Read the model definition and answer for the solid it produces. Units are mm, in the model's axes. A direction names the side the tool comes from. Coordinates: 2 decimals unless noted, no trailing zeros. Write each loop counter-clockwise with the first axis right and the second up, starting at its lowest first coordinate (ties: lowest second). Pieces come first, ordered by that corner, then holes.
Item 1: Straight lines are drawn through the part: probe 1 along X at (y, z) = (2.45, -253); probe 2 along X at (y, z) = (2.3, -255); probe 3 along X at (y, z) = (2.4, -228.5). For each, find the intervals that lie inside material, in ascending order.
Item 2: A tool of negligible diameter and unlimited length cuts with its end or side. For faces 4 (the face through (252.034, 2, -201)), 5 (the face through (247, 3.175, -240)), from which of +Z, -Z, +X, -X, +Y, -Y can it reach the whole face along a straight path? Write none if from no direction.
Item 3: Determine the mould class of faces 1 (the face through (240, 2, -269.211)), 2 (the face through (265, 2, -193.011)), 3 (the face through (236.533, 2.976, -253.457)) for opening direction Z: released by +Z, released by -Z, zero draft, split by the parting line, or undercut.
Item 4: Section C-C (x = 230) is taken. Give the vertices of the cut face in (y, z) (3 decimals), then the cut area to 3 significant figures.
Item 5: Section B-B (x = 262) is taken. State how many separate pieces and enclosed holes the cut face has, then the cut area to 3 significant figures.
Item 6: Section A-A (y = 1.35) is taken. Give the vertices of the cut face in (x, z).
Item 7: This flat-tipped pin is pushed along its axis until it touches: P1, Ø8, axis at x = 253.5, z = -215, coming from the -Y side. Where does it stop, or does it pass through?
from build123d import *

# Parameters (mm, degrees)
BOSS_EXTRUDE1_DEPTH                  = 3.175
F_1_4_0_25_DIAMETER_HOLE1_AT_2_COUNT = 2
F_1_4_0_25_DIAMETER_HOLE1_AT_2_PITCH = 25.4
F_1_4_0_25_DIAMETER_HOLE1_AT_3_COUNT = 2
F_1_4_0_25_DIAMETER_HOLE1_AT_3_PITCH = 50.8
F_1_4_0_25_DIAMETER_HOLE1_AT_4_COUNT = 2
F_1_4_0_25_DIAMETER_HOLE1_AT_4_PITCH = 56.796126628
F_1_4_0_25_DIAMETER_HOLE1_AT_5_COUNT = 2
F_1_4_0_25_DIAMETER_HOLE1_AT_5_PITCH = 71.842048969


with BuildPart() as part:
    # Sketch1 → Boss-Extrude1 (new body)
    with BuildSketch(Plane(origin=(0, 0, 0), x_dir=(1, 0, 0), z_dir=(0, 1, 0))):
        with BuildLine():
            Line((274.893771244, 269.21115375), (203.773771244, 269.21115375))
            ThreePointArc((203.773771244, 269.21115375), (201.97772002, 268.467204975), (201.233771244, 266.67115375))
            Line((201.233771244, 266.67115375), (201.233771244, 246.35115375))
            ThreePointArc((201.233771244, 246.35115375), (201.97772002, 244.555102526), (203.773771244, 243.81115375))
            Line((203.773771244, 243.81115375), (213.933771244, 243.81115375))
            ThreePointArc((213.933771244, 243.81115375), (240.874539608, 232.651922114), (252.033771244, 205.71115375))
            Line((252.033771244, 205.71115375), (252.033771244, 195.55115375))
            ThreePointArc((252.033771244, 195.55115375), (252.77772002, 193.755102526), (254.573771244, 193.01115375))
            Line((254.573771244, 193.01115375), (274.893771244, 193.01115375))
            ThreePointArc((274.893771244, 193.01115375), (276.689822469, 193.755102526), (277.433771244, 195.55115375))
            Line((277.433771244, 195.55115375), (277.433771244, 266.67115375))
            ThreePointArc((277.433771244, 266.67115375), (276.689822469, 268.467204975), (274.893771244, 269.21115375))
        make_face()
    extrude(amount=BOSS_EXTRUDE1_DEPTH)

    # Sketch4 → 1/4 (0.25) Diameter Hole1 (revolve, cut)
    with BuildSketch(Plane(origin=(264.733771244, 0, -205.71115375), x_dir=(0, 0, -1), z_dir=(1, 0, 0))):
        Polygon((0, 0), (0, 3.175), (3.175, 3.175), (3.175, 4.090710056), (6.731, 0), align=None)
    f_1_4_0_25_diameter_hole1 = revolve(axis=Axis((264.733771244, -6.35, -205.71115375), (0, 1, 0)), mode=Mode.SUBTRACT)

    # 1/4 (0.25) Diameter Hole1 at 2: 1/4 (0.25) Diameter Hole1 ×2
    with Locations(*[(0, 0, -i * F_1_4_0_25_DIAMETER_HOLE1_AT_2_PITCH) for i in range(1, F_1_4_0_25_DIAMETER_HOLE1_AT_2_COUNT)]):
        add(f_1_4_0_25_diameter_hole1, mode=Mode.SUBTRACT)

    # 1/4 (0.25) Diameter Hole1 at 3: 1/4 (0.25) Diameter Hole1 ×2
    with Locations(*[(0, 0, -i * F_1_4_0_25_DIAMETER_HOLE1_AT_3_PITCH) for i in range(1, F_1_4_0_25_DIAMETER_HOLE1_AT_3_COUNT)]):
        add(f_1_4_0_25_diameter_hole1, mode=Mode.SUBTRACT)

    # 1/4 (0.25) Diameter Hole1 at 4: 1/4 (0.25) Diameter Hole1 ×2
    with Locations(*[Vector(-0.44721359549993195, 0, -0.894427190999929) * (i * F_1_4_0_25_DIAMETER_HOLE1_AT_4_PITCH) for i in range(1, F_1_4_0_25_DIAMETER_HOLE1_AT_4_COUNT)]):
        add(f_1_4_0_25_diameter_hole1, mode=Mode.SUBTRACT)

    # 1/4 (0.25) Diameter Hole1 at 5: 1/4 (0.25) Diameter Hole1 ×2
    with Locations(*[Vector(-0.7071067811865277, 0, -0.7071067811865673) * (i * F_1_4_0_25_DIAMETER_HOLE1_AT_5_PITCH) for i in range(1, F_1_4_0_25_DIAMETER_HOLE1_AT_5_COUNT)]):
        add(f_1_4_0_25_diameter_hole1, mode=Mode.SUBTRACT)


solid = part.part
Established:
1. probe 1: x = 201.23 to 210.96, 216.91 to 236.36, 242.31 to 261.76, 267.71 to 277.43
1. probe 2: x = 201.23 to 209.45, 218.42 to 234.85, 243.82 to 260.25, 269.22 to 277.43
1. probe 3: x = 244.47 to 260.89, 268.58 to 277.43
2. face 4: +Z, -X, +Y, -Y
2. face 5: +Z, -Z, +X, -X, +Y
3. face 1: released by -Z
3. face 2: released by +Z
3. face 3: undercut
4. outline: (0, -269.211) - (3.175, -269.211) - (3.175, -240.258) - (0, -240.258) - close
4. area: 91.9 mm2
5. separate pieces: 4
5. enclosed holes: 0
5. area: 155 mm2
6. outline: (201.23, -266.67) arc R2.54 ccw to (203.77, -269.21) - (274.89, -269.21) arc R2.54 ccw to (277.43, -266.67) - (277.43, -195.55) arc R2.54 ccw to (274.89, -193.01) - (254.57, -193.01) arc R2.54 ccw to (252.03, -195.55) - (252.03, -205.71) arc R38.1 cw to (213.93, -243.81) - (203.77, -243.81) arc R2.54 ccw to (201.23, -246.35) - close; hole circle Ø11.11 at (213.93, -256.51); hole circle Ø11.11 at (239.33, -256.51); hole circle Ø11.11 at (264.73, -256.51); hole circle Ø11.11 at (264.73, -231.11); hole circle Ø11.11 at (264.73, -205.71)
7. P1: stops at y = 0
